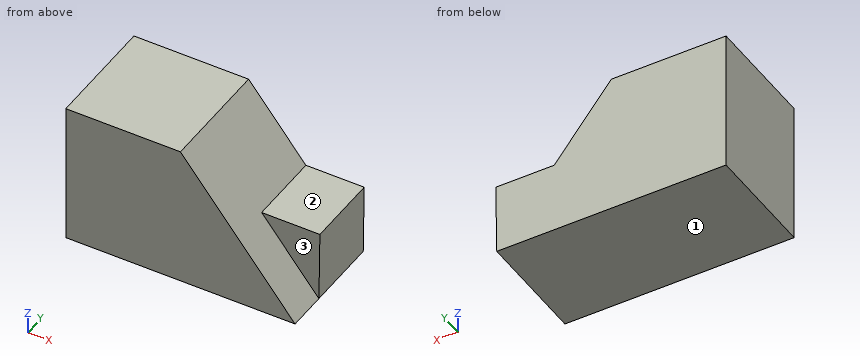
```python
from build123d import *

# Parameters (mm, degrees)
F0_W     = 50.8
F0_H     = 31.75
F1_DEPTH = 25.4
F3_DEPTH = 25.401
F5_DEPTH = 16.51


with BuildPart() as f1:
    # F0 (on Front) → F1 (new body)
    with BuildSketch(Plane.XZ):
        with Locations((-29.731384, 39.01551)):
            Rectangle(F0_W, F0_H)
    extrude(amount=F1_DEPTH)

    # F2 (on face) → F3 (cut, through all)
    with BuildSketch(Plane.XZ.offset(25.4)):
        Polygon((-4.331384, 54.89051), (-29.731384, 54.89051), (-4.331384, 23.14051), align=None)
    extrude(amount=-F3_DEPTH, mode=Mode.SUBTRACT)

    # F4 (on face) → F5 (join)
    with BuildSketch(Plane(origin=(0, 0, 0), x_dir=(-1, 0, 0), z_dir=(0, 1, 0))):
        Polygon((4.331384, 23.14051), (17.031384, 39.01551), (4.114715, 39.01551), align=None)
    extrude(amount=-F5_DEPTH)


solid = f1.part
```
Geometry check sheet. Reference: the model listing, model coordinates, mm. Face numbers are marked on the shaded views. A direction names the side the tool comes from. Round coordinates to 2 decimals unless told otherwise and drop trailing zeros. Order: outer loops, then holes, each group sorted by start corner. A loop starts at its lowest first (then second) coordinate and runs counter-clockwise, first axis right, second up. Notation, with made-up numbers: (-25, -34) - (8, -34) arc R20 ccw to (8, -19) - close; hole circle Ø2 at (46, 49). An arc over 180 degrees is marked (long way). Use a Markdown table: item, result. Add a question column.
1) Thickness scan on line 1 along Z through (x, y) = (-15.5, -4.25); line 2 along X through (y, z) = (-14.5, 44); line 3 along X through (y, z) = (-11.5, 30.5). Record the ranges inside material, lowest first.
2) Set-up check for the marked faces 1, 2 and 3: record each of +Z, -Z, +X, -X, +Y, -Y from which the full face is reachable in a straight line by a thin tool's end or side.
3) Section check B-B (z = 35). Record the cut outline in (x, y), then the cut area to 3 significant figures.
4) Section check C-C (x = -18). Record the cut outline in (y, z).
5) Section check D-D (y = -23.5). Record the cut outline in (x, z).
6) Section check A-A (y = -13.25). Record the cut outline in (x, z).
7) Gauge pin test, flat ends, axial feed: P1, Ø1, axis at x = -9.5, y = -14.5, coming from the +Z side; P2, Ø3, axis at x = -10, y = -21.5, coming from the +Z side. Record the tip position at first contact, or that the pin passes through.
Established:
| question | item | result |
|---|---|---|
| 1 | line 1 | 23.14 to 39.02 |
| 1 | line 2 | -55.13 to -21.02 |
| 1 | line 3 | -55.13 to -4.23 |
| 2 | face 1 | -Z, +X, -X, +Y, -Y |
| 2 | face 2 | +Z, +X, +Y, -Y |
| 2 | face 3 | +Z, +X, -Y |
| 3 | outline | (-55.13, -25.4) - (-13.82, -25.4) - (-13.82, -16.51) - (-4.17, -16.51) - (-4.17, 0) - (-55.13, 0) - close |
| 3 | area | 1,210 mm2 |
| 4 | outline | (-25.4, 23.14) - (0, 23.14) - (0, 40.23) - (-25.4, 40.23) - close |
| 5 | outline | (-55.13, 23.14) - (-4.33, 23.14) - (-29.73, 54.89) - (-55.13, 54.89) - close |
| 6 | outline | (-55.13, 23.14) - (-4.33, 23.14) - (-4.11, 39.02) - (-17.03, 39.02) - (-29.73, 54.89) - (-55.13, 54.89) - close |
| 7 | P1 | z = 39.02 |
| 7 | P2 | z = 32.1 |
